Autodesk Inventor part; units mm, degrees
ref_plane "YZ Plane" through (0, 0, 0) normal (1, 0, 0) x (0, 1, 0)
ref_plane "XZ Plane" through (0, 0, 0) normal (0, 1, 0) x (-1, 0, 0)
ref_plane "XY Plane" through (0, 0, 0) normal (0, 0, 1) x (1, 0, 0)
sketch "Skizze1" plane through (0, 0, 0) normal (0, 1, 0) x (-1, 0, 0)
  line L0 (-17.5, 39) -> (17.5, 39)
  line L1 (17.5, 39) -> (17.5, -39)
  line L2 (17.5, -39) -> (-17.5, -39)
  line L3 (-17.5, -39) -> (-17.5, 39)
  line L4 (-17.5, 39) -> (17.5, -39) construction
  line L5 (17.5, 39) -> (-17.5, -39) construction
  point P0 (0, 0)
  dimension "d0" = 78
  dimension "d1" = 35
extrude "Extrusion1" add sketch "Skizze1" along normal blind 10
sketch "Skizze2" plane through (0, 0, 0) normal (0, -1, 0) x (1, 0, 0)
  line L0 (17.5, 39) -> (-17.5, 39)
  line L1 (-17.5, 39) -> (-17.5, -39)
  line L2 (-17.5, -39) -> (17.5, -39)
  line L3 (17.5, -39) -> (17.5, 39)
  line L4 (17.5, 39) -> (17.5, -39)
  line L5 (-17.5, -14) -> (17.5, -14)
  line L6 (17.5, -14) -> (17.5, 21)
  line L7 (17.5, 21) -> (-17.5, 21)
  line L8 (-17.5, 21) -> (-17.5, -14)
  point P0 (0, 0)
  dimension "d4" = 18
  dimension "d5" = 25
extrude "Extrusion2" add sketch "Skizze2" along normal blind 10 contours L3 L5 L1 L7
sketch "Skizze3" plane through (0, 10, 0) normal (0, 1, 0) x (1, 0, 0)
  line L0 (17.5, -39) -> (17.5, 39)
  line L1 (-17.5, -39) -> (17.5, -39)
  point P0 (0, 0)
  point P1 (2.5, -3.5)
  dimension "d8" = 15
  dimension "d9" = 35.5
hole "Bohrung1" at (2.5, 10, 3.5) direction (0, -1, 0) diameter 6 end through all counterbore diameter 12 counterbore depth 5
chamfer "Fase1" distance 5 angle 45 2 edges at (0, 10, 39) (0, 10, -39)
properties part number "Holding_Plate_Frame" material "PC/ABS-Kunststoff"
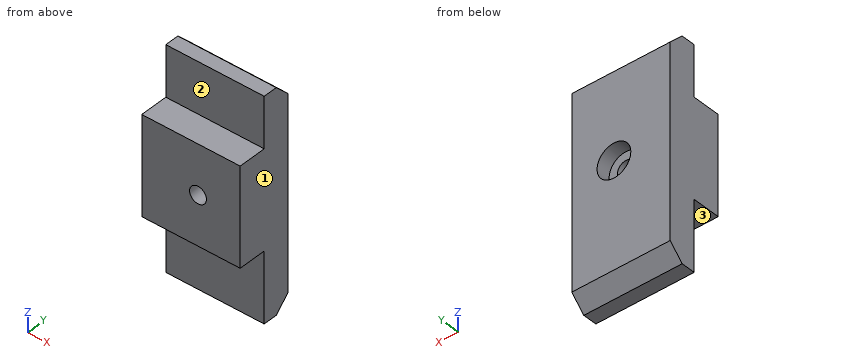
CAD build for the part. Positions are in the model's coordinates, mm. Face numbers are marked on the shaded views. A direction names the side the tool comes from. Give positions to 0.01 mm unless a question says otherwise; leave off trailing zeros. Order: outer loops, then holes, each group sorted by start corner. A loop starts at its lowest first (then second) coordinate and runs counter-clockwise, first axis right, second up.
(1) Drill centre lines: L1, parallel to X at y = 7.7, z = 3.5; L2, parallel to Z at x = 2.5, y = -4; L3, parallel to X at y = -2.25, z = 3.5. Where is each one in solid material? Low to high.
(2) Tool access for the marked faces 1, 2 and 3: list every direction of +Z, -Z, +X, -X, +Y, -Y with a clear straight run to the whole face (end or side of a thin tool).
(3) Saw through at A-A, the plane z = 3.5. Give the cut face in (x, y).
(4) Saw through at C-C, the plane y = -2. Give the cut face in (x, z), then the cut area to 3 significant figures.
(5) Saw through at D-D, the plane x = -12. Give the cut face in (y, z), then the cut area to 4 significant figures.
(6) Saw through at B-B, the plane x = 2.5. Give the cut face in (y, z).
(7) Flat gauge pins, fed straight in: pin 1 (9.5 mm diameter, centred on x = 0, z = 3, fed in from +Y); pin 2 (3 mm diameter, centred on x = -1, y = 7, fed in from +Z); pin 3 (6 mm diameter, centred on x = 12.5, y = -5, fed in from -Z); pin 4 (7.5 mm diameter, centred on x = -3, z = -31.5, fed in from -Y). Where does each tip first touch, or does it go through?
Results found:
1. L1: x = -17.5 to -3.5, 8.5 to 17.5
1. L2: z = -14 to 0.5, 6.5 to 21
1. L3: x = -17.5 to -0.5, 5.5 to 17.5
2. face 1: +Z, -Z, +X, +Y, -Y
2. face 2: +Z, +X, -X, -Y
2. face 3: -Z, +X, -X, -Y
3. outline: (-17.5, -10) - (-0.5, -10) - (-0.5, 5) - (-3.5, 5) - (-3.5, 10) - (-17.5, 10) - close; (5.5, -10) - (17.5, -10) - (17.5, 10) - (8.5, 10) - (8.5, 5) - (5.5, 5) - close
4. outline: (-17.5, -14) - (17.5, -14) - (17.5, 21) - (-17.5, 21) - close; hole circle Ø6 at (2.5, 3.5)
4. area: 1,200 mm2
5. outline: (-10, -14) - (0, -14) - (0, -39) - (5, -39) - (10, -34) - (10, 34) - (5, 39) - (0, 39) - (0, 21) - (-10, 21) - close
5. area: 1,105 mm2
6. outline: (-10, -14) - (0, -14) - (0, -39) - (5, -39) - (10, -34) - (10, -2.5) - (5, -2.5) - (5, 0.5) - (-10, 0.5) - close; (-10, 6.5) - (5, 6.5) - (5, 9.5) - (10, 9.5) - (10, 34) - (5, 39) - (0, 39) - (0, 21) - (-10, 21) - close
7. pin 1: stops at y = 10
7. pin 2: stops at z = 38.5
7. pin 3: stops at z = -14
7. pin 4: stops at y = 0
